The listing builds one solid part. Answer for the finished solid, in the listing's coordinates (mm). Face numbers are marked on the shaded views. A direction names the side the tool comes from. Coordinates: 2 decimals unless noted, no trailing zeros. Write each loop counter-clockwise with the first axis right and the second up, starting at its lowest first coordinate (ties: lowest second). Pieces come first, ordered by that corner, then holes.
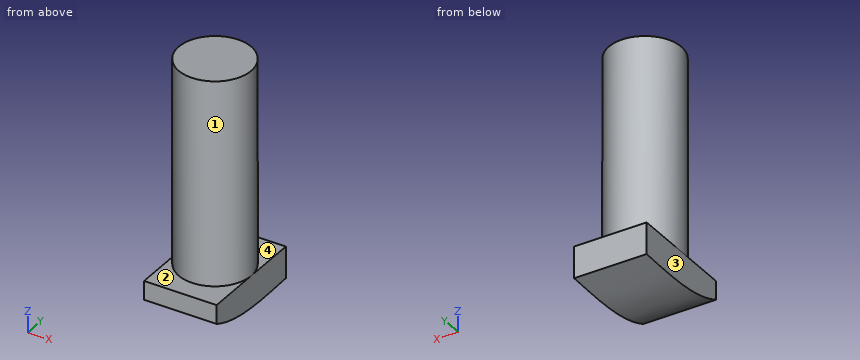
from build123d import *

# Parameters (mm, degrees)
SKETCH1_R           = 2.3
BOSS_EXTRUDE1_DEPTH = 13
SKETCH2_W           = 4.6
SKETCH2_H           = 7
BOSS_EXTRUDE2_DEPTH = 3
CUT_EXTRUDE1_DEPTH  = 4.6


with BuildPart() as part:
    # Sketch1 → Boss-Extrude1 (new body)
    with BuildSketch(Plane.XY):
        with Locations(Location((0, 0, 0), (0, 0, 180))):
            Circle(SKETCH1_R)
    extrude(amount=BOSS_EXTRUDE1_DEPTH)

    # Sketch2 → Boss-Extrude2 (add)
    with BuildSketch(Plane(origin=(0, 0, 0), x_dir=(-1, 0, 0), z_dir=(0, 0, -1))):
        Rectangle(SKETCH2_W, SKETCH2_H)
    extrude(amount=BOSS_EXTRUDE2_DEPTH)

    # Sketch3 → Cut-Extrude1 (cut)
    with BuildSketch(Plane(origin=(2.3, 0, 0), x_dir=(0, 0, -1), z_dir=(1, 0, 0))):
        with BuildLine():
            Line((1.2, -3.5), (3, -3.5))
            Line((3, -3.5), (3, 3.5))
            Line((3, 3.5), (2.011534301, 3.5))
            add(Edge.make_bspline(
                [(1.2, -3.5), (2.267514736, -1.334400874), (2.08240034, 1.182388913), (2.011534301, 3.5)],
                knots=[0, 0, 0, 0, 1, 1, 1, 1], degree=3))
        make_face()
    extrude(amount=-CUT_EXTRUDE1_DEPTH, mode=Mode.SUBTRACT)


solid = part.part
1. Section A-A on z = 9 is taken. Give the vertices of the cut face in (x, y).
Results found:
outline: circle Ø4.6 at (0, 0)
2. Find the intervals of material crossed by L1, parallel to Z at x = 0.1, y = 1; L2, parallel to Y at x = -1.65, z = 8; L3, parallel to Y at x = -1.85, z = 4.75, in increasing order.
Results found:
L1: z = -2.07 to 13
L2: y = -1.6 to 1.6
L3: y = -1.37 to 1.37
3. A tool of negligible diameter and unlimited length cuts with its end or side. For the marked faces 1, 2, 3 and 4, from which of +Z, -Z, +X, -X, +Y, -Y can it reach the whole face along a straight path? Write none if from no direction.
Results found:
face 1: +Z
face 2: +Z, -Y
face 3: +Z, -Z, -X, +Y, -Y
face 4: +Z, +Y
4. Flat-ended cylindrical pins translate along their axes: P1, Ø1, axis at x = 0.5, z = 6, coming from the -Y side; P2, Ø1.5, axis at x = -2, z = 2, coming from the -Y side. Find the tip coordinate at first contact, or state that the pin passes through.
Results found:
P1: stops at y = -2.3
P2: stops at y = -1.93
